from build123d import *

# Parameters (mm, degrees)
F1_DEPTH = 5
F3_DEPTH = 25
F5_DEPTH = 25


with BuildPart() as f1:
    # F0 (on Top) → F1 (new body)
    with BuildSketch(Plane.XY):
        with BuildLine():
            ThreePointArc((4.3541757575, 0), (9.7452402115, 5.391064454), (15.1363046655, 0))
            Line((15.1363046655, 0), (18.3717107881, 0))
            ThreePointArc((18.3717107881, 0), (9.7452402115, 8.6264705766), (1.1187696349, 0))
            Line((1.1187696349, 0), (4.3541757575, 0))
        make_face()
        with BuildLine():
            Line((18.3717107881, 0), (15.1363046655, 0))
            ThreePointArc((15.1363046655, 0), (9.7452402115, -5.391064454), (4.3541757575, 0))
            Line((4.3541757575, 0), (1.1187696349, 0))
            ThreePointArc((1.1187696349, 0), (7.678470178, -8.3752287275), (17.3813779901, -4.0131526802))
            ThreePointArc((17.3813779901, -4.0131526802), (18.1204689389, -2.0667700335), (18.3717107881, 0))
        make_face()
        with BuildLine():
            Line((19.490480423, 0), (18.3717107881, 0))
            ThreePointArc((18.3717107881, 0), (18.1204689389, -2.0667700335), (17.3813779901, -4.0131526802))
            Line((17.3813779901, -4.0131526802), (19.490480423, 0))
        make_face()
        with BuildLine():
            ThreePointArc((17.3813779901, -4.0131526802), (7.678470178, -8.3752287275), (1.1187696349, 0))
            Line((1.1187696349, 0), (0, 0))
            Line((0, 0), (-9.5463581383, -18.164595589))
            Line((-9.5463581383, -18.164595589), (-2.7843534481, -35.9314270318))
            Line((-2.7843534481, -35.9314270318), (-11.0048279166, -56.8803735077))
            Line((-11.0048279166, -56.8803735077), (3.0495305546, -49.9857850373))
            Line((3.0495305546, -49.9857850373), (14.1869476065, -35.9314270318))
            Line((14.1869476065, -35.9314270318), (9.9441222847, -18.164595589))
            Line((9.9441222847, -18.164595589), (17.3813779901, -4.0131526802))
        make_face()
        with BuildLine():
            ThreePointArc((4.3541757575, 0), (9.7452402115, -5.391064454), (15.1363046655, 0))
            Line((15.1363046655, 0), (4.3541757575, 0))
        make_face()
    extrude(amount=F1_DEPTH)

    # F2 (on face) → F3 (cut)
    with BuildSketch(Plane.XY.offset(5)):
        Polygon((1.1187696349, -24.7765574604), (0, 0), (-1.0323523379, -1.9643368131), (0, -24.8270747891), align=None)
        Polygon((10.3103312495, -19.6980956646), (9.9441222847, -18.164595589), (0, -34.1810695827), (0.9515207789, -34.7718387486), align=None)
    extrude(amount=-F3_DEPTH, mode=Mode.SUBTRACT)

    # F4 (on face) → F5 (cut)
    with BuildSketch(Plane.XY.offset(5)):
        Polygon((3.6861358676, -8.3900917694), (6.1861358676, -8.3900917694), (6.1861358676, -13.3900917694), (7.1861358676, -13.3900917694), (7.1861358676, -8.3900917694), (9.6861358676, -8.3900917694), (9.6861358676, -7.3900917694), (9.0056210756, -7.3900917694), (3.6861358676, -7.3900917694), align=None)
    extrude(amount=-F5_DEPTH, mode=Mode.SUBTRACT)


solid = f1.part
Input: part model. Units: mm. Frame: model coordinates. A direction names the side the tool comes from. Give positions to 0.01 mm unless a question says otherwise; leave off trailing zeros. Order: outer loops, then holes, each group sorted by start corner. A loop starts at its lowest first (then second) coordinate and runs counter-clockwise, first axis right, second up. Notation, with made-up numbers: (-35.5, -40) -> (-19.5, -40) arc R22 ccw to (-19.5, -8) -> close; hole circle Ø9 at (34, 68.25). An arc over 180 degrees is marked (long way). Use one line per item in the form item = value.
1) Section A-A, the plane z = 2.65. Return loops of the section in (x, y), and give its area (3 significant figures).
Response values:
outline = (-11, -56.88) -> (3.05, -49.99) -> (14.19, -35.93) -> (10.31, -19.7) -> (0.95, -34.77) -> (0, -34.18) -> (9.94, -18.16) -> (19.49, 0) -> (18.37, 0) arc R8.63 ccw to (1.12, 0) -> (0, 0) -> (1.12, -24.78) -> (0, -24.83) -> (-1.03, -1.96) -> (-9.55, -18.16) -> (-2.78, -35.93) -> close; hole (3.69, -8.39) -> (6.19, -8.39) -> (6.19, -13.39) -> (7.19, -13.39) -> (7.19, -8.39) -> (9.69, -8.39) -> (9.69, -7.39) -> (3.69, -7.39) -> close; hole (4.35, 0) -> (15.14, 0) arc R5.39 ccw to start
area = 929 mm^2
2) Line query: probe 1 along Y at (x, z) = (5.5, 4.7); probe 2 along Y at (x, z) = (10, 1.4); probe 3 along Y at (x, z) = (8.5, 4.25). Output: solid intervals per line, ascending.
Response values:
probe_1 = -46.89 to -27.45, -25.32 to -8.39, -7.39 to 0, 3.32 to 7.51
probe_2 = -41.21 to -20.2, -18.06 to 0, 5.39 to 8.62
probe_3 = -43.11 to -22.61, -20.49 to -8.39, -7.39 to 0, 5.25 to 8.54
3) Section B-B, the plane x = 13. Return loops of the section in (y, z).
Response values:
outline = (-37.43, 0) -> (-30.96, 0) -> (-30.96, 5) -> (-37.43, 5) -> close; (-12.35, 0) -> (0, 0) -> (0, 5) -> (-12.35, 5) -> close; (4.3, 0) -> (7.99, 0) -> (7.99, 5) -> (4.3, 5) -> close
4) Section D-D, the plane y = -42.5. Return loops of the section in (x, z).
Response values:
outline = (-5.36, 0) -> (8.98, 0) -> (8.98, 5) -> (-5.36, 5) -> close
5) First-contact query: pin 1 Ø0.6 at (x, z) = (19, 3) entering from +Y; pin 2 Ø2.5 at (x, z) = (8, 2) entering from +Y; pin 3 Ø2 at (y, z) = (-33.5, 1) entering from -X. Flat tips, straight axial feed; report the tip coordinate or a pass-through.
Response values:
pin_1 = 0
pin_2 = 8.61
pin_3 = -4.09
6) Reachability of faces 1 (the flat face through (4, -24, 0)), 2 (the flat face through (0.6, 0, 2.5)), 3 (the flat face through (0.6, -24.8, 2.5)), 4 (the flat face through (12.276, -27.928, 2.465)) from +Z, -Z, +X, -X, +Y, -Y: full face, straight path, thin tool, end or side. Return the list, or none.
Response values:
face_1 = -Z, +X, -X, +Y, -Y
face_2 = +Z, -Z, -X, +Y
face_3 = +Z, -Z
face_4 = +Z, -Z, +X
7) Section C-C, the plane y = -3. Return loops of the section in (x, z).
Response values:
outline = (-1.58, 0) -> (-0.99, 0) -> (-0.99, 5) -> (-1.58, 5) -> close; (0.14, 0) -> (17.91, 0) -> (17.91, 5) -> (0.14, 5) -> close
8) Mould query, pull axis X, two halves, no side actions, for faces 5 (the flat face through (4, -24, 5)), 6 (the flat face through (-6.213, -26.924, 2.465)), 7 (the flat face through (-4.076, -53.481, 2.465)), 8 (the flat face through (10, 0, 2)). Classes: pulls with the +X half, pulls with the -X half, needs draft (parallel to the pull), parting line crosses it, or undercut.
Response values:
face_5 = needs draft
face_6 = pulls with the -X half
face_7 = pulls with the +X half
face_8 = undercut
